```python
from build123d import *

# Parameters (mm, degrees)
F0_R     = 13.6
F0_R_2   = 10.95
F1_DEPTH = 7


with BuildPart() as f1:
    # F0 (on Top) → F1 (new body)
    with BuildSketch(Plane.XY):
        Circle(F0_R)
        Circle(F0_R_2, mode=Mode.SUBTRACT)
    extrude(amount=F1_DEPTH)

    # F2 (on Front) → F3 (revolve, cut)
    with BuildSketch(Plane.XZ):
        Polygon((13.6, 3.59), (13.6, 6.39), (11.85, 5.379637), (11.85, 4.600363), align=None)
    revolve(axis=Axis((0, 0, 7), (0, 0, 1)), mode=Mode.SUBTRACT)


solid = f1.part
```
The listing builds one solid part. Answer for the finished solid, in the listing's coordinates (mm). Coordinates: 2 decimals unless noted, no trailing zeros. Loops run counter-clockwise (first coordinate to the right, second up) from the corner with the lowest first, then second, coordinate; pieces in that order, holes last. Notation, with made-up numbers: (-13.5, 15.5) -> (22.5, 15.5) arc R16 ccw to (22.5, 24.5) -> close; hole circle Ø3 at (19.25, 3.5). An arc over 180 degrees is marked (long way). Return JSON: item names as keys, results as strings. Group by question number.
(1) Find the intervals of material crossed by probe 1 along Y at (x, z) = (0, 3); probe 2 along Y at (x, z) = (0, 4.75); probe 3 along Z at (x, y) = (-11.25, 5), in increasing order. Write a range as from..to.
(2) A cutting plane is placed at C-C on z = 5. Write down the section's boundary in (x, y).
(3) Determine the mould class of faces 1 (the cylindrical face through (11.303, 3.559, 4.985)), 2 (the flat face through (0.9, 11.1, 0)), 3 (the cylindrical face through (-8.69, -6.66, 3.45)) for opening direction Y: released by +Y, released by -Y, zero draft, split by the parting line, or undercut.
(4) A cutting plane is placed at A-A on x = 0. Write down the section's boundary in (y, z).
(5) Given pin 1 Ø2 at (x, z) = (6.5, 5.5) entering from -Y; pin 2 Ø1.5 at (y, z) = (7.5, 5) entering from +X, each flat-ended and moving along its own axis, determine where each tip first touches the part or whether it passes through.
The answers:
{
 "1": {"probe 1": "y = -13.6..-10.95, 10.95..13.6", "probe 2": "y = -11.85..-10.95, 10.95..11.85", "probe 3": "z = 0..4.33, 5.65..7"},
 "2": {"outline": "circle Ø23.7 at (0, 0); hole circle Ø21.9 at (0, 0)"},
 "3": {"face 1": "split by the parting line", "face 2": "zero draft", "face 3": "undercut"},
 "4": {"outline": "(-13.6, 0) -> (-10.95, 0) -> (-10.95, 7) -> (-13.6, 7) -> (-13.6, 6.39) -> (-11.85, 5.38) -> (-11.85, 4.6) -> (-13.6, 3.59) -> close; (10.95, 0) -> (13.6, 0) -> (13.6, 3.59) -> (11.85, 4.6) -> (11.85, 5.38) -> (13.6, 6.39) -> (13.6, 7) -> (10.95, 7) -> close"},
 "5": {"pin 1": "stops at y = -12.18", "pin 2": "stops at x = 10.08"}
}
